Build history of the part. All positions in model axes, mm. Face numbers are marked on the shaded views. A direction names the side the tool comes from. Round coordinates to 2 decimals unless told otherwise and drop trailing zeros. Write each loop counter-clockwise with the first axis right and the second up, starting at its lowest first coordinate (ties: lowest second). Pieces come first, ordered by that corner, then holes. Notation, with made-up numbers: (42, 18) -> (51, 18) arc R34 ccw to (51, 48) -> close; hole circle Ø9 at (46.25, 13). An arc over 180 degrees is marked (long way). One line per question, with ' | ' between items.
from build123d import *

# Parameters (mm, degrees)
F0_W     = 19
F0_H     = 50
F1_DEPTH = 16
F2_W     = 13.5
F2_H     = 13.5011018194
F3_DEPTH = 50
F4_W     = 100
F4_H     = 16
F4_W_2   = 13.2999992773
F4_H_2   = 13.4999992773
F4_W_3   = 10.3
F4_H_3   = 10.5
F5_DEPTH = 2.75
F6_DEPTH = 15


with BuildPart() as f1:
    # F0 (on Top) → F1 (new body)
    with BuildSketch(Plane.XY):
        Rectangle(F0_W, F0_H)
    extrude(amount=F1_DEPTH)

    # F2 (on face) → F3 (cut)
    with BuildSketch(Plane.XZ.offset(25)):
        with Locations((0, 6.7505509097)):
            Rectangle(F2_W, F2_H)
    extrude(amount=-F3_DEPTH, mode=Mode.SUBTRACT)

    # F4 (on face) → F5 (join)
    with BuildSketch(Plane.YZ.offset(9.5)):
        with Locations((0, 8)):
            Rectangle(F4_W, F4_H)
        with Locations((-40.3361745238, 7.9659550227)):
            Rectangle(F4_W_2, F4_H_2, mode=Mode.SUBTRACT)
        with Locations((40.3361745238, 7.9659550227)):
            Rectangle(F4_W_2, F4_H_2, mode=Mode.SUBTRACT)
        with Locations((-40.3361745238, 7.9659550227)):
            Rectangle(F4_W_2, F4_H_2)
        with Locations((-40.3361745238, 7.9659550227)):
            Rectangle(F4_W_3, F4_H_3, mode=Mode.SUBTRACT)
        with Locations((40.3361745238, 7.9659550227)):
            Rectangle(F4_W_2, F4_H_2)
        with Locations((40.3361745238, 7.9659550227)):
            Rectangle(F4_W_3, F4_H_3, mode=Mode.SUBTRACT)
        with Locations((-40.3361745238, 7.9659550227)):
            Rectangle(F4_W_3, F4_H_3)
        with Locations((40.3361745238, 7.9659550227)):
            Rectangle(F4_W_3, F4_H_3)
    extrude(amount=-F5_DEPTH)

    # F4 (on face) → F6 (join)
    with BuildSketch(Plane.YZ.offset(9.5)):
        with Locations((-40.3361745238, 7.9659550227)):
            Rectangle(F4_W_2, F4_H_2)
        with Locations((-40.3361745238, 7.9659550227)):
            Rectangle(F4_W_3, F4_H_3, mode=Mode.SUBTRACT)
        with Locations((40.3361745238, 7.9659550227)):
            Rectangle(F4_W_2, F4_H_2)
        with Locations((40.3361745238, 7.9659550227)):
            Rectangle(F4_W_3, F4_H_3, mode=Mode.SUBTRACT)
    extrude(amount=F6_DEPTH)


solid = f1.part
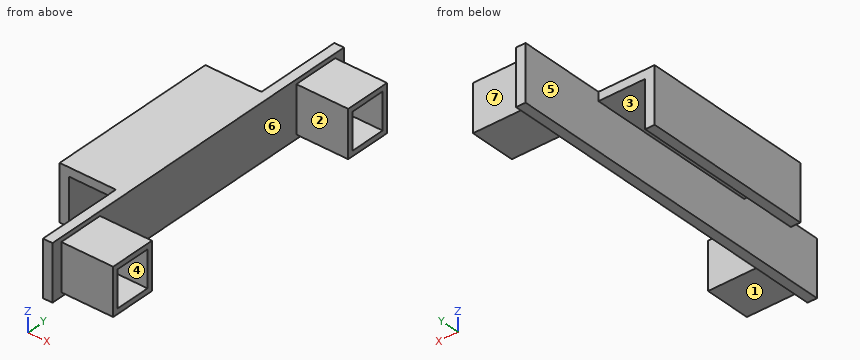
(1) Slice it at D-D (x = 0.5). Write the cut outline in (y, z).
Calculated:
outline: (-25, 13.5) -> (25, 13.5) -> (25, 16) -> (-25, 16) -> close
(2) 3-axis set-ups, long thin cutter, end or side, ignore diameter. For the marked faces 1, 2, 3 and 4: which of +Z, -Z, +X, -X, +Y, -Y reach the whole face in a straight line?
Calculated:
face 1: -Z, +X, +Y, -Y | face 2: +Z, -Z, +X | face 3: -Z, +Y, -Y | face 4: +X
(3) Slice it at A-A (x = 21). Write the cut outline in (y, z), then the cut area to 3 significant figures.
Calculated:
outline: (-46.99, 1.22) -> (-33.69, 1.22) -> (-33.69, 14.72) -> (-46.99, 14.72) -> close; (33.69, 1.22) -> (46.99, 1.22) -> (46.99, 14.72) -> (33.69, 14.72) -> close; hole (-45.49, 2.72) -> (-35.19, 2.72) -> (-35.19, 13.22) -> (-45.49, 13.22) -> close; hole (35.19, 2.72) -> (45.49, 2.72) -> (45.49, 13.22) -> (35.19, 13.22) -> close | area: 143 mm2
(4) Wall check: line 1 (Y direction, x = 20.5, z = 14.5); line 2 (X direction, y = -10, z = 12.5); line 3 (Z direction, x = -6, y = -17). Give the ranges that are in metal, low to high. Write a range as from..to.
Calculated:
line 1: -46.99..-33.69, 33.69..46.99 | line 2: -9.5..-6.75, 6.75..9.5 | line 3: 13.5..16
(5) Mould opens along Y. For the marked faces 5, 6 and 7 say: pulls with the +Y half, pulls with the -Y half, needs draft (parallel to the pull), parting line crosses it, or undercut.
Calculated:
face 5: needs draft | face 6: undercut | face 7: pulls with the +Y half
(6) Slice it at B-B (z = 12.25). Write the cut outline in (x, y), then the cut area to 4 significant figures.
Calculated:
outline: (-9.5, -25) -> (-6.75, -25) -> (-6.75, 25) -> (-9.5, 25) -> close; (6.75, -50) -> (9.5, -50) -> (9.5, -46.99) -> (24.5, -46.99) -> (24.5, -45.49) -> (9.5, -45.49) -> (9.5, -35.19) -> (24.5, -35.19) -> (24.5, -33.69) -> (9.5, -33.69) -> (9.5, 33.69) -> (24.5, 33.69) -> (24.5, 35.19) -> (9.5, 35.19) -> (9.5, 45.49) -> (24.5, 45.49) -> (24.5, 46.99) -> (9.5, 46.99) -> (9.5, 50) -> (6.75, 50) -> close | area: 502.5 mm2
(7) Drop flat-ended pins along their axis: pin 1 (10 mm diameter, centred on x = -1, y = -13, fed in from -Z); pin 2 (6.5 mm diameter, centred on x = 20, z = 10.5, fed in from -Y); pin 3 (11.5 mm diameter, centred on x = 17, y = 42.5, fed in from -Z). Give the stop position or say it passes through.
Calculated:
pin 1: z = 13.5 | pin 2: y = -46.99 | pin 3: z = 1.22
(8) Slice it at C-C (y = -5.5). Write the cut outline in (x, z).
Calculated:
outline: (-9.5, 0) -> (-6.75, 0) -> (-6.75, 13.5) -> (6.75, 13.5) -> (6.75, 0) -> (9.5, 0) -> (9.5, 16) -> (-9.5, 16) -> close
